Could you check a few things on this model? Use its own coordinates, in mm. Face numbers are marked on the shaded views. Coordinates: 2 decimals unless noted, no trailing zeros. Write each loop counter-clockwise with the first axis right and the second up, starting at its lowest first coordinate (ties: lowest second). Pieces come first, ordered by that corner, then holes.
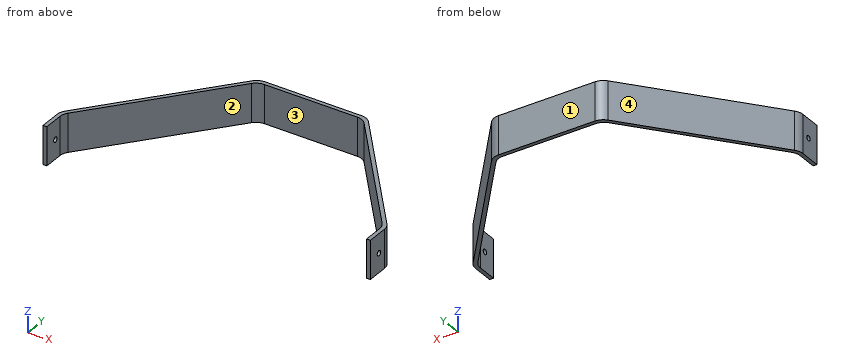
```python
from build123d import *

# Parameters (mm, degrees)
BOSS_EXTRUDE1_DEPTH     = 30
FILLET1_R               = 10
CUT_EXTRUDE1_DEPTH      = 287.462912085
CUT_EXTRUDE1_DEPTH_BACK = 287.462912085
SKETCH2_R               = 2


with BuildPart() as part:
    # Sketch1 → Boss-Extrude1 (new body)
    with BuildSketch(Plane.XY):
        Polygon((128, -125), (125, -125), (125, -106.066937462), (41.07406521, -3), (-41.07406521, -3), (-125, -106.066937462), (-125, -125), (-128, -125), (-128, -105), (-42.5, 0), (42.5, 0), (128, -105), align=None)
    extrude(amount=BOSS_EXTRUDE1_DEPTH)

    # Fillet1
    fillet1_edges = [part.edges().sort_by_distance(p)[0] for p in [
        (125, -106.066937462, 15),
        (41.07406521, -3, 15),
        (-41.07406521, -3, 15),
        (-125, -106.066937462, 15),
        (-128, -105, 15),
        (-42.5, 0, 15),
        (42.5, 0, 15),
        (128, -105, 15),
    ]]
    fillet(fillet1_edges, radius=FILLET1_R)

    # Sketch2 → Cut-Extrude1 (cut, two sides: drawn at the far end of the back side and taken through both)
    with BuildSketch(Plane(origin=(128, 0, 0), x_dir=(0, 0, -1), z_dir=(1, 0, 0)).offset(-CUT_EXTRUDE1_DEPTH_BACK)):
        with Locations((-15, -115)):
            Circle(SKETCH2_R)
    extrude(amount=CUT_EXTRUDE1_DEPTH + CUT_EXTRUDE1_DEPTH_BACK, mode=Mode.SUBTRACT)


solid = part.part
```
1. For pin 1 (1 mm diameter, centred on x = 74, z = 19, fed in from +Y); pin 2 (4 mm diameter, centred on y = -91.5, z = 8.5, fed in from +X); pin 3 (5 mm diameter, centred on y = -39.5, z = 14, fed in from -X), each with a flat end and sliding along its axis, tell me the tip position at first contact or that it passes through.
Verdict:
pin 1: stops at y = -38.07
pin 2: stops at x = 118.64
pin 3: stops at x = -76.7
2. Please list where these lines run through material, in increasing order: line 1 along Z through (x, y) = (126, -115); line 2 along X through (y, z) = (-42.5, 24.25); line 3 along Y through (x, z) = (126.65, 15).
Verdict:
line 1: z = 0 to 13, 17 to 30
line 2: x = -77.11 to -73.24, 73.24 to 77.11
line 3: y = -125 to -117, -113 to -103.54
3. If we mould it in two halves opening along X, with no side actions, what happens to the marked faces 1, 2, 3 and 4? For each: pulls with the +X half, pulls with the -X half, needs draft (parallel to the pull), parting line crosses it, or undercut.
Verdict:
face 1: needs draft
face 2: undercut
face 3: undercut
face 4: pulls with the -X half
4. I want a section at C-C on x = -81.5. Please give me the cut outline in (y, z).
Verdict:
outline: (-52.65, 0) - (-47.89, 0) - (-47.89, 30) - (-52.65, 30) - close
5. I want a section at B-B on z = 19.75. Please give me the cut outline in (x, y), plus the area to 3 significant figures.
Verdict:
outline: (-128, -125) - (-125, -125) - (-125, -109.62) arc R10 cw to (-122.75, -103.31) - (-44.08, -6.69) arc R10 cw to (-36.32, -3) - (36.32, -3) arc R10 cw to (44.08, -6.69) - (122.75, -103.31) arc R10 cw to (125, -109.62) - (125, -125) - (128, -125) - (128, -108.56) arc R10 ccw to (125.75, -102.24) - (45.5, -3.69) arc R10 ccw to (37.75, 0) - (-37.75, 0) arc R10 ccw to (-45.5, -3.69) - (-125.75, -102.24) arc R10 ccw to (-128, -108.56) - close
area: 1,170 mm2
6. I want a section at A-A on y = -80.5. Please give me the cut outline in (x, z).
Verdict:
outline: (-108.05, 0) - (-104.18, 0) - (-104.18, 30) - (-108.05, 30) - close; (104.18, 0) - (108.05, 0) - (108.05, 30) - (104.18, 30) - close
